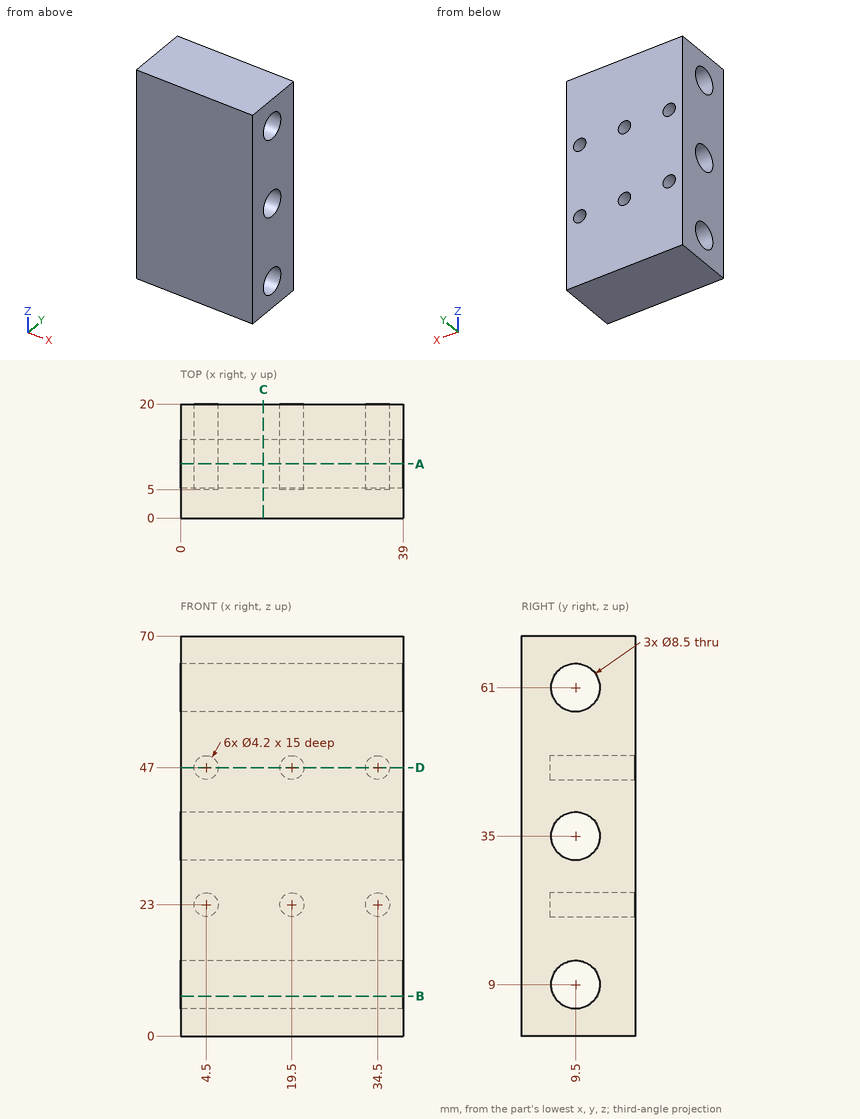
Input: dimensioned drawing with shaded views. Units: mm. Origin: part minimum x, y, z. Give positions to 0.01 mm unless a question says otherwise; leave off trailing zeros. Order: outer loops, then holes, each group sorted by start corner. A loop starts at its lowest first (then second) coordinate and runs counter-clockwise, first axis right, second up.
(1) Section query D-D (z = 47). Return the cut outline in (x, y).
(2) Material intervals for line 1 along X through (y, z) = (16.5, 23); line 2 along Y through (x, z) = (10, 35); line 3 along Z through (x, y) = (6, 13), sorted ascending.
(3) Section query B-B (z = 7). Return the cut outline in (x, y), plus the area to 4 significant figures.
(4) Contact query for flat-ended pins moving along their axis: P1, Ø6.5, axis at x = 4.5, z = 47, coming from the -Y side; P2, Ø4, axis at x = 19.5, z = 47, coming from the +Y side. Output: stop coordinate, or through.
(5) Section query C-C (x = 14.5). Return the cut outline in (y, z), plus the area to 3 significant figures.
(6) Section query A-A (y = 9.5). State how many separate pieces and enclosed holes the cut face has, plus the area to 3 significant figures.
Outcome:
1. outline: (0, 0) - (39, 0) - (39, 20) - (36.6, 20) - (36.6, 5) - (32.4, 5) - (32.4, 20) - (21.6, 20) - (21.6, 5) - (17.4, 5) - (17.4, 20) - (6.6, 20) - (6.6, 5) - (2.4, 5) - (2.4, 20) - (0, 20) - close
2. line 1: x = 0 to 2.4, 6.6 to 17.4, 21.6 to 32.4, 36.6 to 39
2. line 2: y = 0 to 5.25, 13.75 to 20
2. line 3: z = 0 to 6.59, 11.41 to 21.53, 24.47 to 32.59, 37.41 to 45.53, 48.47 to 58.59, 63.41 to 70
3. outline: (0, 0) - (39, 0) - (39, 5.75) - (0, 5.75) - close; (0, 13.25) - (39, 13.25) - (39, 20) - (0, 20) - close
3. area: 487.5 mm2
4. P1: stops at y = 0
4. P2: stops at y = 5
5. outline: (0, 0) - (20, 0) - (20, 70) - (0, 70) - close; hole circle Ø8.5 at (9.5, 9); hole circle Ø8.5 at (9.5, 35); hole circle Ø8.5 at (9.5, 61)
5. area: 1,230 mm2
6. separate pieces: 4
6. enclosed holes: 6
6. area: 1,650 mm2
